The model under review builds one solid part; all positions refer to its coordinate system, in mm. Face numbers are marked on the shaded views. A direction names the side the tool comes from. Round coordinates to 2 decimals unless told otherwise and drop trailing zeros. Order: outer loops, then holes, each group sorted by start corner. A loop starts at its lowest first (then second) coordinate and runs counter-clockwise, first axis right, second up. Notation, with made-up numbers: M 33.25,47 L 75.25,47 A5 cw 75.25,56 Z; hole C 75.5,-23 d1. An arc over 180 degrees is marked long. Use a Markdown table: item, result. Add a question column.
1. Consider section D-D on x = -92.5. State the section outline as (y, z) points, then the cut area to 3 significant figures.
2. To check wall thickness, follow probe 1 along Z at (x, y) = (-16.5, 50.5); probe 2 along Y at (x, z) = (-170, 105); probe 3 along Y at (x, z) = (-181, 14). State the ranges of each line that lie inside material, in increasing order.
3. For the marked faces 1, 2, 3, 4 and 5, list the 3-axis set-ups (+Z, -Z, +X, -X, +Y, -Y) from which the entire face can be reached by the end or side of a thin tool; tool diameter is ignored.
4. The part is to be moulded in two halves that separate along Y. For the marked faces 6, 7 and 8, say which applies: +Y half, -Y half, draft (parallel to the pull), parting line (faces both ways), or undercut.
5. Consider section A-A on z = 16.5. State the section outline as (x, y) points.
6. Consider section C-C on y = 69. State the section outline as (x, z) points.
7. Consider section B-B on x = -154. State the section outline as (y, z) points.
8. Insertion check: P1, Ø12, axis at y = 66.5, z = 79.5, coming from the +X side; P2, Ø12, axis at x = -90.5, z = 36.5, coming from the -Y side; P3, Ø6, axis at y = 337.5, z = 84, coming from the +X side. Each pin has a flat end and moves straight along its axis. Give the tip position at first contact, or say it passes through.
from build123d import *

# Parameters (mm, degrees)
BOSS_EXTRUDE1_DEPTH = 116.84
FILLET1_R           = 50.8
SHELL2_T            = -2.54


with BuildPart() as part:
    # Sketch1 → Boss-Extrude1 (new body)
    with BuildSketch(Plane.XY):
        Polygon((0, 0), (0, 266.7), (-63.5, 355.6), (-279.4, 482.6), (-279.4, 177.8), (-63.5, 88.9), align=None)
    extrude(amount=BOSS_EXTRUDE1_DEPTH)

    # Fillet1
    fillet1_edges = [part.edges().sort_by_distance(p)[0] for p in [
        (-63.5, 88.9, 58.42),
        (-63.5, 355.6, 58.42),
    ]]
    fillet(fillet1_edges, radius=FILLET1_R)

    # Shell2
    shell2_openings = [part.faces().sort_by_distance(p)[0] for p in [
        (-279.4, 330.2, 58.42),
        (0, 133.35, 58.42),
    ]]
    offset(amount=SHELL2_T, openings=shell2_openings, kind=Kind.INTERSECTION)


solid = part.part
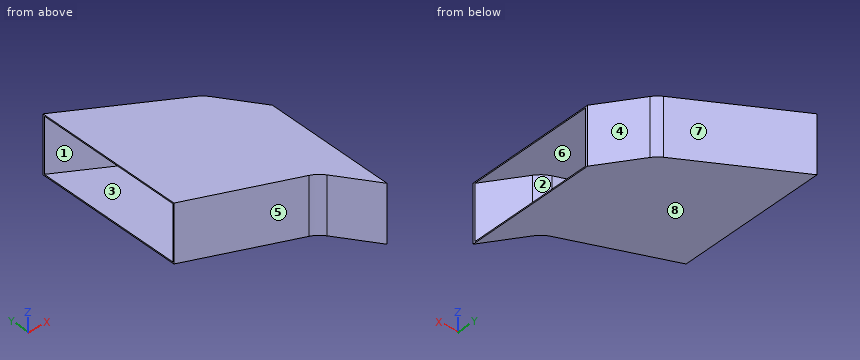
Answer block:
| question | item | result |
|---|---|---|
| 1 | outline | M 100.84,0 L 372.66,0 L 372.66,116.84 L 100.84,116.84 Z; hole M 103.59,2.54 L 369.71,2.54 L 369.71,114.3 L 103.59,114.3 Z |
| 1 | area | 2,020 mm^2 |
| 2 | probe 1 | 0 to 2.54, 114.3 to 116.84 |
| 2 | probe 2 | 132.75 to 135.5, 415.3 to 418.25 |
| 2 | probe 3 | 137.28 to 140.03, 421.77 to 424.72 |
| 3 | face 1 | -X |
| 3 | face 2 | +X |
| 3 | face 3 | none |
| 3 | face 4 | +Z, -Z, +X, +Y |
| 3 | face 5 | +Z, -Z, -X, -Y |
| 4 | face 6 | undercut |
| 4 | face 7 | +Y half |
| 4 | face 8 | draft |
| 5 | outline | M -279.4,177.8 L -77.01,94.46 A50.8 cw -55.01,77.01 L 0,0 L 0,4.37 L -52.94,78.49 A53.34 ccw -76.04,96.81 L -279.4,180.55 Z; M -279.4,479.65 L -74.09,358.88 A48.26 cw -59.29,345.34 L 0,262.33 L 0,266.7 L -57.22,346.81 A50.8 ccw -72.81,361.07 L -279.4,482.6 Z |
| 6 | outline | M -49.29,0 L 0,0 L 0,2.54 L -46.16,2.54 L -46.16,114.3 L 0,114.3 L 0,116.84 L -49.29,116.84 Z |
| 7 | outline | M 126.16,0 L 408.84,0 L 408.84,116.84 L 126.16,116.84 Z; hole M 128.91,2.54 L 405.89,2.54 L 405.89,114.3 L 128.91,114.3 Z |
| 8 | P1 | x = -40.09 |
| 8 | P2 | y = 97.55 |
| 8 | P3 | x = -48.43 |
